```python
from build123d import *

# Parameters (mm, degrees)
F1_DEPTH      = 4.445
F2_W          = 47.752
F2_H          = 63.5
F3_DEPTH      = 9.398
F5_DEPTH      = 47.752
F7_DEPTH      = 17.2212
F7_DEPTH_BACK = 17.2212
F8_R          = 1.27


with BuildPart() as f1:
    # F0 (on Top) → F1 (new body)
    with BuildSketch(Plane.XY):
        with BuildLine():
            Line((-24.003, -39.8145), (24.003, -39.8145))
            ThreePointArc((24.003, -39.8145), (25.350038, -39.256538), (25.908, -37.9095))
            Line((25.908, -37.9095), (25.908, 37.9095))
            ThreePointArc((25.908, 37.9095), (25.350038, 39.256538), (24.003, 39.8145))
            Line((24.003, 39.8145), (-24.003, 39.8145))
            ThreePointArc((-24.003, 39.8145), (-25.350038, 39.256538), (-25.908, 37.9095))
            Line((-25.908, 37.9095), (-25.908, -37.9095))
            ThreePointArc((-25.908, -37.9095), (-25.350038, -39.256538), (-24.003, -39.8145))
        make_face()
    extrude(amount=F1_DEPTH)

    # F2 (on face) → F3 (join)
    with BuildSketch(Plane(origin=(0, 0, 0), x_dir=(1, 0, 0), z_dir=(0, 0, -1))):
        Rectangle(F2_W, F2_H)
    extrude(amount=F3_DEPTH)

    # F4 (on face) → F5 (join, through all)
    with BuildSketch(Plane(origin=(-23.876, 0, 0), x_dir=(0, -1, 0), z_dir=(-1, 0, 0))):
        with BuildLine():
            Line((-34.29, -9.398), (-31.75, -9.398))
            Line((-31.75, -9.398), (-31.75, -5.461))
            Line((-31.75, -5.461), (-33.655, -5.461))
            ThreePointArc((-33.655, -5.461), (-34.104013, -5.646987), (-34.29, -6.096))
            Line((-34.29, -6.096), (-34.29, -9.398))
        make_face()
        with BuildLine():
            ThreePointArc((34.29, -6.096), (34.104013, -5.646987), (33.655, -5.461))
            Line((33.655, -5.461), (31.75, -5.461))
            Line((31.75, -5.461), (31.75, -9.398))
            Line((31.75, -9.398), (34.29, -9.398))
            Line((34.29, -9.398), (34.29, -6.096))
        make_face()
    extrude(amount=-F5_DEPTH)

    # F6 (on Front) → F7 (join, two sides)
    with BuildSketch(Plane.XZ) as f7_sk:
        Polygon((-30.861, -9.398), (-23.876, -9.398), (-23.876, 0), (-25.908, 0), (-30.861, -8.128), align=None)
        Polygon((30.861, -9.398), (30.861, -8.128), (25.908, 0), (23.876, 0), (23.876, -9.398), align=None)
    extrude(amount=F7_DEPTH)
    extrude(f7_sk.sketch, amount=-F7_DEPTH_BACK)

    # F8
    f8_edges = [f1.edges().sort_by_distance(p)[0] for p in [
        (23.876, -17.2212, -4.699),
        (23.876, 17.2212, -4.699),
        (-23.876, 17.2212, -4.699),
        (-23.876, -17.2212, -4.699),
    ]]
    fillet(f8_edges, radius=F8_R)


solid = f1.part
```
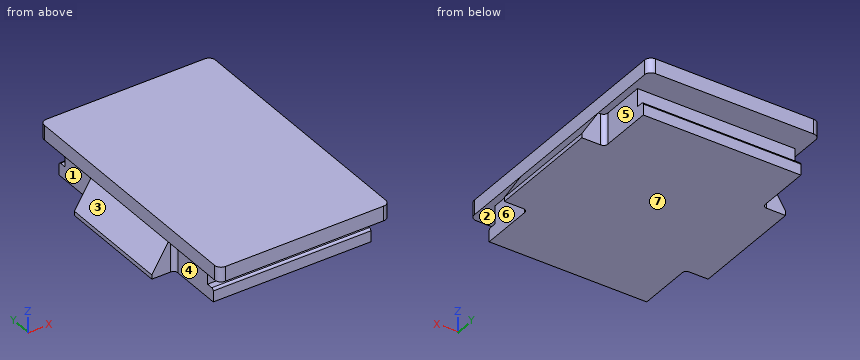
The listing builds one solid part. Answer for the finished solid, in the listing's coordinates (mm). Face numbers are marked on the shaded views. A direction names the side the tool comes from. Give positions to 0.01 mm unless a question says otherwise; leave off trailing zeros. Loops run counter-clockwise (first coordinate to the right, second up) from the corner with the lowest first, then second, coordinate; pieces in that order, holes last. Notation, with made-up numbers: (25, 82.5) - (70, 82.5) arc R20 cw to (70, 87.5) - close; hole circle Ø1 at (45, 39). An arc over 180 degrees is marked (long way). Answer as CSV lines item,"result". Start each with the question number.
Item 1: For the marked faces 4, 5, 6 and 7, determine the directions among +Z, -Z, +X, -X, +Y, -Y from which every point of the face is accessible in a straight line to the end or side of a thin tool.
Item 2: A cutting plane is placed at D-D on z = -3.5. Determine the outline of the cut face in (x, y).
Item 3: Find the intervals of material crossed by line 1 (Y direction, x = 7.5, z = -6.5); line 2 (X direction, y = 31, z = -6.25); line 3 (Y direction, x = -11.5, z = -1), in increasing order. Write a range as from..to.
Item 4: A cutting plane is placed at A-A on y = -16. Determine the outline of the cut face in (x, z) (3 decimals).
Item 5: A cutting plane is placed at C-C on z = 2.25. Determine the outline of the cut face in (x, y) (1 decimal).
Item 6: The mould has two halves that part along Z. Classify the marked faces 1, 2 and 3: +Z half, -Z half, draft (parallel to the pull), parting line (faces both ways), or undercut.
Item 7: Each of these flat-tipped pins is pushed along its axis until it touches: pin 1 (2 mm diameter, centred on y = -9.5, z = 2.5, fed in from -X); pin 2 (4.5 mm diameter, centred on y = 29.5, z = -2.5, fed in from -X); pin 3 (2.5 mm diameter, centred on x = 11, z = -8.5, fed in from +Y). Where does it stop, or does it pass through?
Found:
1,face 4,"-Z, -X, -Y"
1,face 5,"-Z, +X, +Y"
1,face 6,"-Z, +X, -Y"
1,face 7,"-Z, +X, -X, +Y, -Y"
2,outline,"(-28.04, -17.22) - (-25.15, -17.22) arc R1.27 cw to (-23.88, -18.49) - (-23.88, -31.75) - (23.88, -31.75) - (23.88, -18.49) arc R1.27 cw to (25.15, -17.22) - (28.04, -17.22) - (28.04, 17.22) - (25.15, 17.22) arc R1.27 cw to (23.88, 18.49) - (23.88, 31.75) - (-23.88, 31.75) - (-23.88, 18.49) arc R1.27 cw to (-25.15, 17.22) - (-28.04, 17.22) - close"
3,line 1,"y = -34.29..34.29"
3,line 2,"x = -23.88..23.88"
3,line 3,"y = -31.75..31.75"
4,outline,"(-30.861, -9.398) - (30.861, -9.398) - (30.861, -8.128) - (25.908, 0) - (25.908, 4.445) - (-25.908, 4.445) - (-25.908, 0) - (-30.861, -8.128) - close"
5,outline,"(-25.9, -37.9) arc R1.9 ccw to (-24, -39.8) - (24, -39.8) arc R1.9 ccw to (25.9, -37.9) - (25.9, 37.9) arc R1.9 ccw to (24, 39.8) - (-24, 39.8) arc R1.9 ccw to (-25.9, 37.9) - close"
6,face 1,"draft"
6,face 2,"undercut"
6,face 3,"+Z half"
7,pin 1,"stops at x = -25.91"
7,pin 2,"stops at x = -23.88"
7,pin 3,"stops at y = 34.29"
